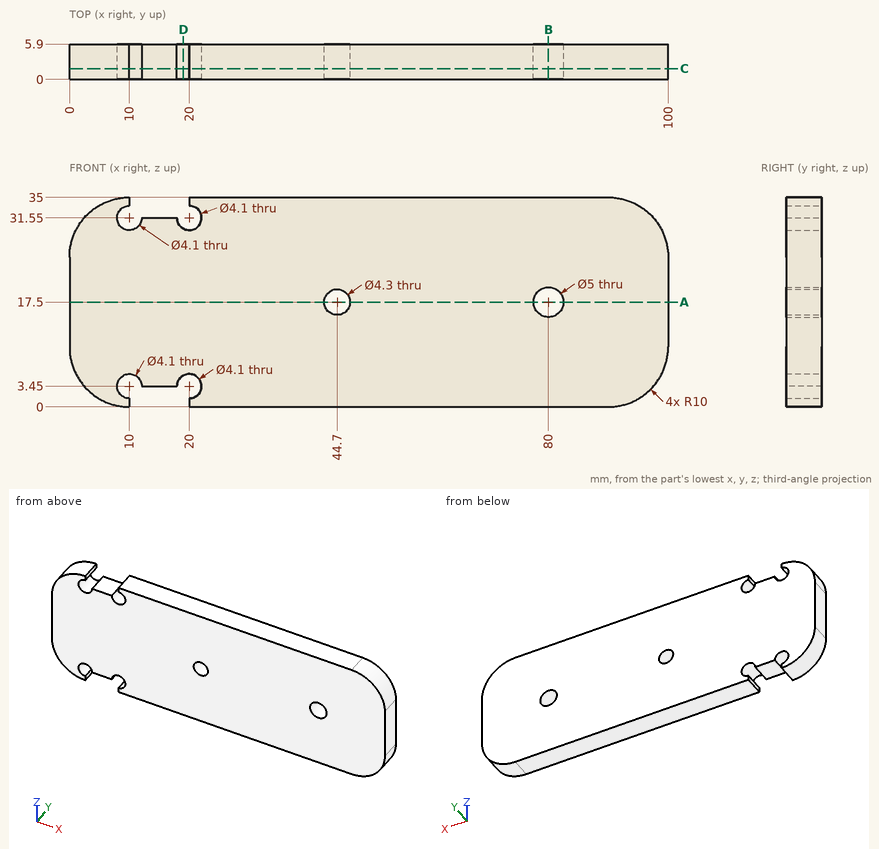
Here's the drawing with two shaded views (mm, measured from the low corner). I have some questions. Round coordinates to 2 decimals unless told otherwise and drop trailing zeros. Write each loop counter-clockwise with the first axis right and the second up, starting at its lowest first coordinate (ties: lowest second). Pieces come first, ordered by that corner, then holes. Notation, with made-up numbers: M 34,57.5 L 83,57.5 A11 ccw 83,63.5 Z; hole C -21,36.5 d4. An arc over 180 degrees is marked long. Answer in a Markdown table with one row per item. Add a question column.
Q1. Imagine slicing it at A-A (z = 17.5). Please give me the cut outline in (x, y), then the cut area to 3 significant figures.
Q2. Will these pins go through, and if not, where does the flat tip stop? pin 1 Ø1.1 at (y, z) = (4, 0.5) entering from +X; pin 2 Ø4 at (x, z) = (80, 17.5) entering from +Y; pin 3 Ø1.5 at (y, z) = (4, 34.5) entering from +X; pin 4 Ø3 at (x, y) = (14, 2.5) entering from +Z.
Q3. Imagine slicing it at D-D (x = 19). Please give me the cut outline in (y, z), then the cut area to 3 significant figures.
Q4. Imagine slicing it at C-C (y = 1.8). Please give me the cut outline in (x, z).
Q5. Imagine slicing it at B-B (x = 80). Please give me the cut outline in (y, z).
Q6. If I drill on line 1 (X direction, y = 4.05, z = 17.5); line 2 (X direction, y = 2.7, z = 3.5); line 3 (Z direction, x = 44.7, y = 2.6), over which ranges is the centre line in solid material (lowest first)? Write a range as from..to.
Values:
| question | item | result |
|---|---|---|
| 1 | outline | M 0,0 L 42.55,0 L 42.55,5.9 L 0,5.9 Z; M 46.85,0 L 77.5,0 L 77.5,5.9 L 46.85,5.9 Z; M 82.5,0 L 100,0 L 100,5.9 L 82.5,5.9 Z |
| 1 | area | 535 mm^2 |
| 2 | pin 1 | x = 94.46 |
| 2 | pin 2 | through |
| 2 | pin 3 | x = 94.84 |
| 2 | pin 4 | z = 31.55 |
| 3 | outline | M 0,5.24 L 5.9,5.24 L 5.9,29.76 L 0,29.76 Z |
| 3 | area | 145 mm^2 |
| 4 | outline | M 0,10 A10 ccw 10,0 L 10,1.4 A2.05 cw long 12.05,3.45 L 17.95,3.45 A2.05 cw long 20,1.4 L 20,0 L 90,0 A10 ccw 100,10 L 100,25 A10 ccw 90,35 L 20,35 L 20,33.6 A2.05 cw long 17.95,31.55 L 12.05,31.55 A2.05 cw long 10,33.6 L 10,35 A10 ccw 0,25 Z; hole C 44.7,17.5 d4.3; hole C 80,17.5 d5 |
| 5 | outline | M 0,0 L 5.9,0 L 5.9,15 L 0,15 Z; M 0,20 L 5.9,20 L 5.9,35 L 0,35 Z |
| 6 | line 1 | 0..42.55, 46.85..77.5, 82.5..100 |
| 6 | line 2 | 2.4..7.95, 12.05..17.95, 22.05..97.6 |
| 6 | line 3 | 0..15.35, 19.65..35 |
